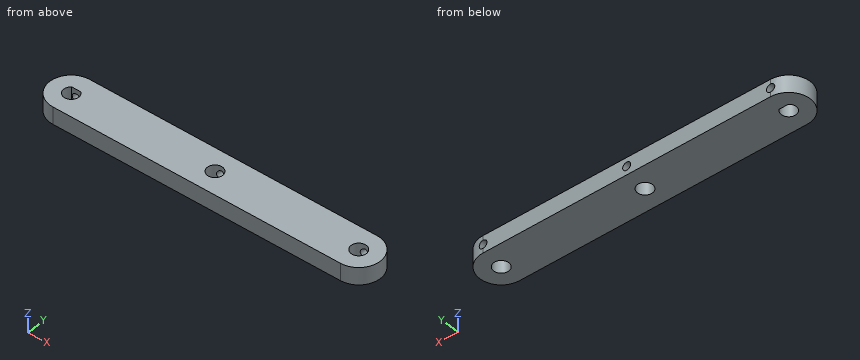
```python
from build123d import *

# Parameters (mm, degrees)
SKETCH1_R           = 2.65
BOSS_EXTRUDE1_DEPTH = 6
CUT_EXTRUDE1_REACH  = 110.707
SKETCH2_R           = 1.4


with BuildPart() as part:
    # Sketch1 → Boss-Extrude1 (new body)
    with BuildSketch(Plane.XY):
        with BuildLine():
            Line((0, 7.5), (100, 7.5))
            ThreePointArc((100, 7.5), (107.5, 0), (100, -7.5))
            Line((100, -7.5), (0, -7.5))
            ThreePointArc((0, -7.5), (-7.5, 0), (0, 7.5))
        make_face()
        with Locations((50, 0)):
            Circle(SKETCH1_R, mode=Mode.SUBTRACT)
        with Locations((100, 0)):
            Circle(SKETCH1_R, mode=Mode.SUBTRACT)
        with BuildLine():
            Line((-1.599218559, 2.05), (1.599218559, 2.05))
            ThreePointArc((1.599218559, 2.05), (0, -2.6), (-1.599218559, 2.05))
        make_face(mode=Mode.SUBTRACT)
    extrude(amount=BOSS_EXTRUDE1_DEPTH)

    # Sketch2 → Cut-Extrude1 (cut, up to next)
    with BuildSketch(Plane(origin=(0, 7.5, 0), x_dir=(1, 0, 0), z_dir=(0, 1, 0)), mode=Mode.PRIVATE) as cut_extrude1_sk1:
        with Locations(Location((0, -3, 0), (0, 0, 90))):
            Circle(SKETCH2_R)
    cut_extrude1_tool1 = extrude(cut_extrude1_sk1.sketch, amount=-CUT_EXTRUDE1_REACH, mode=Mode.PRIVATE) & part.part
    # Sketch2 → Cut-Extrude1 (cut, up to next)
    with BuildSketch(Plane(origin=(0, 7.5, 0), x_dir=(1, 0, 0), z_dir=(0, 1, 0)), mode=Mode.PRIVATE) as cut_extrude1_sk2:
        with Locations(Location((50, -3, 0), (0, 0, 270))):
            Circle(SKETCH2_R)
    cut_extrude1_tool2 = extrude(cut_extrude1_sk2.sketch, amount=-CUT_EXTRUDE1_REACH, mode=Mode.PRIVATE) & part.part
    # Sketch2 → Cut-Extrude1 (cut, up to next)
    with BuildSketch(Plane(origin=(0, 7.5, 0), x_dir=(1, 0, 0), z_dir=(0, 1, 0)), mode=Mode.PRIVATE) as cut_extrude1_sk3:
        with Locations(Location((100, -3, 0), (0, 0, 270))):
            Circle(SKETCH2_R)
    cut_extrude1_tool3 = extrude(cut_extrude1_sk3.sketch, amount=-CUT_EXTRUDE1_REACH, mode=Mode.PRIVATE) & part.part
    add(cut_extrude1_tool1.solids().sort_by_distance((0, 7.5, 3))[0], mode=Mode.SUBTRACT)
    add(cut_extrude1_tool2.solids().sort_by_distance((50, 7.5, 3))[0], mode=Mode.SUBTRACT)
    add(cut_extrude1_tool3.solids().sort_by_distance((100, 7.5, 3))[0], mode=Mode.SUBTRACT)


solid = part.part
```
Check sheet for the modelled part. Datum: model origin and axes. Units: mm. Round coordinates to 2 decimals unless told otherwise and drop trailing zeros. Loops run counter-clockwise (first coordinate to the right, second up) from the corner with the lowest first, then second, coordinate; pieces in that order, holes last. Notation, with made-up numbers: M 34,56 L 92,56 A25 ccw 92,91 Z; hole C 65,89.5 d9. An arc over 180 degrees is marked long. Answer as a JSON object with one key per item and string values.
1. Section check D-D (z = 2.75). Record the boundary of the cut face in (x, y), plus the area to 3 significant figures.
Reply:
{"outline": "M -1.6,2.05 L -1.38,2.05 L -1.38,7.37 A7.5 ccw 0,-7.5 L 100,-7.5 A7.5 ccw 101.38,7.37 L 101.38,2.26 A2.65 cw long 98.62,2.26 L 98.62,7.5 L 51.38,7.5 L 51.38,2.26 A2.65 cw long 48.62,2.26 L 48.62,7.5 L 1.38,7.5 L 1.38,2.05 L 1.6,2.05 A2.6 cw long Z", "area": "1,570 mm²"}
2. Gauge pin test, flat ends, axial feed: P1, Ø1.5, axis at y = -1.5, z = 3.5, coming from the -X side; P2, Ø3, axis at y = -4, z = 3, coming from the -X side; P3, Ø1, axis at y = 2.5, z = 0.5, coming from the +X side. Record the tip position at first contact, or that the pin passes through.
Reply:
{"P1": "stops at x = -7.46", "P2": "stops at x = -7.07", "P3": "stops at x = 107.23"}
3. Section check C-C (y = 6.5). Record the boundary of the cut face in (x, z), plus the area to 3 significant figures.
Reply:
{"outline": "M -3.74,0 L 103.74,0 L 103.74,6 L -3.74,6 Z; hole C 0,3 d2.8; hole C 50,3 d2.8; hole C 100,3 d2.8", "area": "626 mm²"}
4. Section check B-B (x = 50). Record the boundary of the cut face in (y, z).
Reply:
{"outline": "M -7.5,0 L -2.65,0 L -2.65,6 L -7.5,6 Z; M 2.65,0 L 7.5,0 L 7.5,1.6 L 2.65,1.6 Z; M 2.65,4.4 L 7.5,4.4 L 7.5,6 L 2.65,6 Z"}
5. Section check A-A (y = 0). Record the boundary of the cut face in (x, z), plus the area to 3 significant figures.
Reply:
{"outline": "M -7.5,0 L -2.6,0 L -2.6,6 L -7.5,6 Z; M 2.6,0 L 47.35,0 L 47.35,6 L 2.6,6 Z; M 52.65,0 L 97.35,0 L 97.35,6 L 52.65,6 Z; M 102.65,0 L 107.5,0 L 107.5,6 L 102.65,6 Z", "area": "595 mm²"}
6. Scan lines: line 1 (X direction, y = -1.5, z = 3.5); line 2 (Y direction, x = 50, z = 4.75); line 3 (Z direction, x = 50, y = 5.7). Record each from-to range of solid material in increasing order.
Reply:
{"line 1": "x = -7.35 to -2.12, 2.12 to 47.82, 52.18 to 97.82, 102.18 to 107.35", "line 2": "y = -7.5 to -2.65, 2.65 to 7.5", "line 3": "z = 0 to 1.6, 4.4 to 6"}
